```python
from build123d import *

# Parameters (mm, degrees)
EXTRUDE023_DEPTH = 2
CHAMFER001_SIZE  = 2


with BuildPart() as doorlockmountplatecutout:
    # Sketch029 → Extrude023 (new body)
    with BuildSketch(Plane(origin=(0, 0, 0), x_dir=(-1, 0, 0), z_dir=(0, 1, 0))):
        with BuildLine():
            Line((6, 25), (6, -25))
            ThreePointArc((-6, -25), (0, -31), (6, -25))
            Line((-6, -25), (-6, 25))
            ThreePointArc((6, 25), (0, 31), (-6, 25))
        make_face()
    extrude(amount=EXTRUDE023_DEPTH)


with BuildPart() as doorlockmountplatecutout_1:
    # Extrude023 placement: moved
    add(doorlockmountplatecutout.part.moved(Location((170, -55, 0))))


with BuildPart() as mainbody:
    # Sweep: sweep along a path in Sketch001
    with BuildLine(Plane.XZ) as sweep_path:
        ThreePointArc((180, 200), (0, 380), (-180, 200))
        Line((-180, 200), (-180, -200))
        ThreePointArc((-180, -200), (0, -380), (180, -200))
        Line((180, -200), (180, 200))
    # Sketch → Sweep (sweep)
    with BuildSketch(Plane.XY):
        Polygon((160, -55), (160, 35), (170, 35), (170, 55), (180, 55), (180, -55), align=None)
    sweep(path=sweep_path.line)

    # Cut001: cut DoorLockMountPlateCutout
    add(doorlockmountplatecutout_1.part, mode=Mode.SUBTRACT)

    # Chamfer001
    chamfer001_edges = [mainbody.edges().sort_by_distance(p)[0] for p in [
        (0, -55, 380),
        (180, -55, 0),
        (-180, -55, 0),
        (0, -55, -380),
    ]]
    chamfer(chamfer001_edges, length=CHAMFER001_SIZE)


solid = mainbody.part
```
Input: part model. Units: mm. Frame: model coordinates. A direction names the side the tool comes from. Give positions to 0.01 mm unless a question says otherwise; leave off trailing zeros. Order: outer loops, then holes, each group sorted by start corner. A loop starts at its lowest first (then second) coordinate and runs counter-clockwise, first axis right, second up. Notation, with made-up numbers: M 24,78.25 L 65,78.25 A25 cw 65,106.25 Z; hole C -7,78.5 d8. An arc over 180 degrees is marked long. One line per question, with ' | ' between items.
1) Draft query along Z for faces 4 (the face through (3.958, 1.756, 379.956)), 5 (the face through (170, 45, 3)), 6 (the face through (-3.74, 44.86, -369.96)), 7 (the face through (-3.917, -54.875, -378.082)). Return one class per face: pulls with the +Z half, pulls with the -Z half, needs draft (parallel to the pull), parting line crosses it, or undercut.
Filled in:
face 4: pulls with the +Z half | face 5: undercut | face 6: undercut | face 7: pulls with the -Z half
2) Section C-C on y = -40. Output: boundary loops of the cut face in (x, z), and give its area (3 significant figures).
Filled in:
outline: M -180,-200 A180 ccw 180,-200 L 180,200 A180 ccw -180,200 Z; hole M -160,-200 A160 ccw 160,-200 L 160,200 A160 ccw -160,200 Z | area: 37,400 mm2
3) Access query for faces 1 (the face through (-3.958, 1.756, -379.956)), 2 (the face through (-163, 35, -2)), 3 (the face through (3.52, -10.63, 359.96)). Directions: +Z, -Z, +X, -X, +Y, -Y. A direction counts if a zero-diameter tool reaches every point of the face in a straight line with its end or side. Return the directions, or none.
Filled in:
face 1: -Z, +Y, -Y | face 2: +Y | face 3: +Y, -Y
4) Section A-A on x = 0. Output: boundary loops of the cut face in (y, z), and give its area (3 significant figures).
Filled in:
outline: M -55,-378 L -53,-380 L 55,-380 L 55,-370 L 35,-370 L 35,-360 L -55,-360 Z; M -55,360 L 35,360 L 35,370 L 55,370 L 55,380 L -53,380 L -55,378 Z | area: 4,000 mm2
5) Ray query, L1, parallel to X at y = 18.5, z = 159.5; L2, parallel to X at y = 46, z = -68; L3, parallel to Z at x = 33, y = 45. Return the intervals inside material, ascending.
Filled in:
L1: x = -180 to -160, 160 to 180 | L2: x = -180 to -170, 170 to 180 | L3: z = -376.95 to -366.77, 366.77 to 376.95
6) Section B-B on z = -71. Output: boundary loops of the cut face in (x, y).
Filled in:
outline: M -180,-53 L -178,-55 L -160,-55 L -160,35 L -170,35 L -170,55 L -180,55 Z; M 160,-55 L 178,-55 L 180,-53 L 180,55 L 170,55 L 170,35 L 160,35 Z
7) Contact query for flat-ended pins moving along their axis: P1, Ø6, axis at x = 91.5, y = -34.5, coming from the +Z side; P2, Ø1, axis at x = -26, y = 2.5, coming from the -Z side; P3, Ø4, axis at x = -24, y = -40, coming from the +Z side. Output: stop coordinate, or through.
Filled in:
P1: stops at z = 356.74 | P2: stops at z = -378.18 | P3: stops at z = 378.65
